Answer from the drawing. Dimensions are ordinates in mm from the lowest x, y and z of the part. A direction names the side the tool comes from. Coordinates: 2 decimals unless noted, no trailing zeros. Loops run counter-clockwise (first coordinate to the right, second up) from the corner with the lowest first, then second, coordinate; pieces in that order, holes last. Notation, with made-up numbers: (82.25, -39) - (103.25, -39) arc R28 cw to (103.25, -10) - close; hole circle Ø5 at (79.25, 73.5). An arc over 180 degrees is marked (long way). One line per question, with ' | ' between items. Start each with the question number.
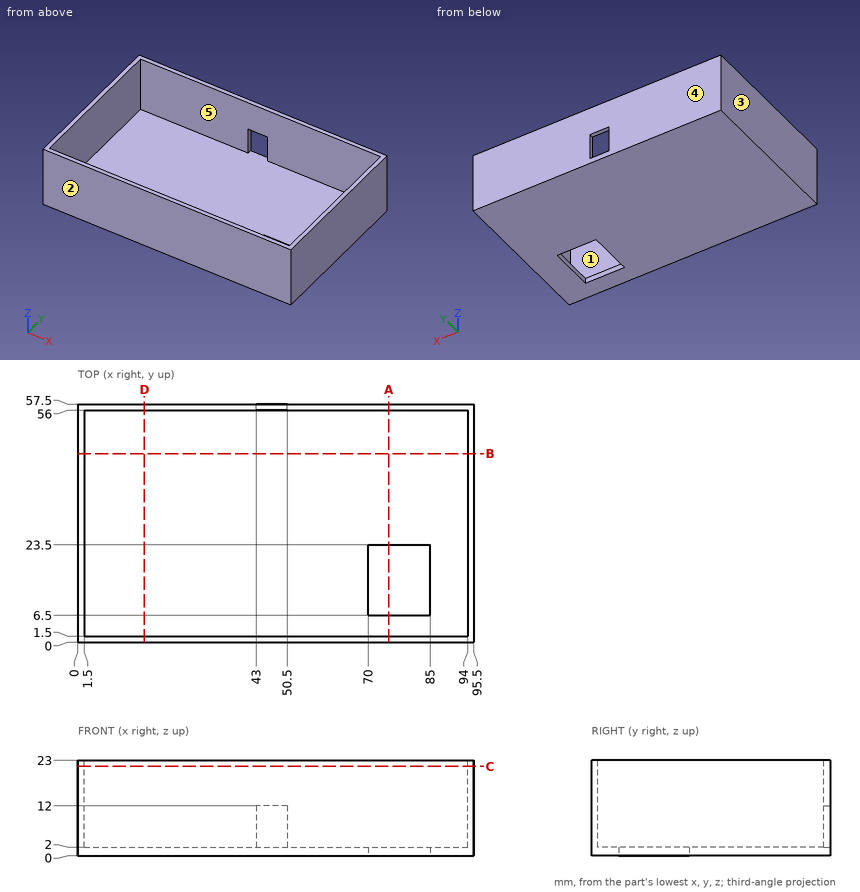
1) The mould has two halves that part along X. Classify the marked faces 1, 2 and 3: released by +X, released by -X, zero draft, split by the parting line, or undercut.
2) The part is cut by section A-A on x = 75. Write down the section's boundary in (y, z), and give its area (3 significant figures).
3) The part is cut by section D-D on x = 16. Write down the section's boundary in (y, z).
4) Find the intervals of material crossed by line 1 along X through (y, z) = (46.5, 9.25); line 2 along Y through (x, z) = (84, 18); line 3 along Z through (x, y) = (15, 34), in increasing order. Write a range as from..to.
5) Given pin 1 Ø2 at (x, y) = (43.5, 37.5) entering from +Z, flat-ended and moving along its own axis, determine where the tip first touches the part or whether it passes through.
6) Which of the six approach directions +Z, -Z, +X, -X, +Y, -Y give full straight-line access (tool end or side, diameter ignored) to the marked faces 4 and 5?
7) The part is cut by section C-C on z = 21.5. Write down the section's boundary in (x, y), and give its area (3 significant figures).
8) The part is cut by section B-B on y = 45.5. Write down the section's boundary in (x, z), and give its area (3 significant figures).
Answer below:
1) face 1: undercut | face 2: zero draft | face 3: released by -X
2) outline: (0, 0) - (6.5, 0) - (6.5, 2) - (1.5, 2) - (1.5, 23) - (0, 23) - close; (23.5, 0) - (57.5, 0) - (57.5, 23) - (56, 23) - (56, 2) - (23.5, 2) - close | area: 144 mm2
3) outline: (0, 0) - (57.5, 0) - (57.5, 23) - (56, 23) - (56, 2) - (1.5, 2) - (1.5, 23) - (0, 23) - close
4) line 1: 0..1.5, 94..95.5 | line 2: 0..1.5, 56..57.5 | line 3: 0..2
5) pin 1: z = 2
6) face 4: +Z, -Z, +X, -X, +Y | face 5: +Z
7) outline: (0, 0) - (95.5, 0) - (95.5, 57.5) - (0, 57.5) - close; hole (1.5, 1.5) - (94, 1.5) - (94, 56) - (1.5, 56) - close | area: 450 mm2
8) outline: (0, 0) - (95.5, 0) - (95.5, 23) - (94, 23) - (94, 2) - (1.5, 2) - (1.5, 23) - (0, 23) - close | area: 254 mm2
